```python
from build123d import *

# Parameters (mm, degrees)
BOSS_EXTRUDE1_OUTLINE_W = 13.462
BOSS_EXTRUDE1_OUTLINE_H = 19.685
BOSS_EXTRUDE1_OUTLINE_R = 2.159
BOSS_EXTRUDE1_DEPTH     = 2.54
SKETCH2_W               = 12.7
SKETCH2_H               = 19.685
SKETCH2_R               = 2.159
BOSS_EXTRUDE2_DEPTH     = 2.54
BOSS_EXTRUDE3_DEPTH     = 12.7
SKETCH4_R               = 1.9685
BOSS_EXTRUDE4_DEPTH     = 1.524


# Read off the part's stored shape, not the designer's step: Boss-Extrude1
with BuildPart() as part:
    # Boss-Extrude1 outline → Boss-Extrude1 (new body)
    with BuildSketch(Plane(origin=(0, 2.413, 0), x_dir=(1, 0, 0), z_dir=(0, 1, 0))):
        with Locations((-28.0035, 0)):
            Rectangle(BOSS_EXTRUDE1_OUTLINE_W, BOSS_EXTRUDE1_OUTLINE_H)
        with Locations((-24.511, -4.7625)):
            Circle(BOSS_EXTRUDE1_OUTLINE_R, mode=Mode.SUBTRACT)
        with Locations((-24.511, 4.7625)):
            Circle(BOSS_EXTRUDE1_OUTLINE_R, mode=Mode.SUBTRACT)
    extrude(amount=BOSS_EXTRUDE1_DEPTH)



with BuildPart() as body_2:
    # Sketch2 → Boss-Extrude2 (new body)
    with BuildSketch(Plane.XZ):
        with Locations((28.3845, 0)):
            Rectangle(SKETCH2_W, SKETCH2_H)
        with Locations(Location((24.511, 4.7625, 0), (0, 0, 270))):
            Circle(SKETCH2_R, mode=Mode.SUBTRACT)
        with Locations(Location((24.511, -4.7625, 0), (0, 0, 270))):
            Circle(SKETCH2_R, mode=Mode.SUBTRACT)
    extrude(amount=BOSS_EXTRUDE2_DEPTH)


with BuildPart() as part_1:
    add(part.part)

    add(body_2.part)  # Boss-Extrude3 merges body 2
    # Sketch3 → Boss-Extrude3 (add, symmetric)
    with BuildSketch(Plane.XY):
        Polygon((34.7345, -2.54), (34.7345, -30.988), (-34.7345, -30.988), (-34.7345, 2.413), (-32.1945, 2.413), (-32.1945, -28.448), (32.1945, -28.448), (32.1945, -2.54), align=None)
        Polygon((-32.1945, 4.953), (-32.1945, 26.884), (33.000418385, 26.884), (33.000418385, 29.424), (-34.7345, 29.424), (-34.7345, 4.953), align=None)
    extrude(amount=BOSS_EXTRUDE3_DEPTH, both=True)

    # Sketch4 → Boss-Extrude4 (add)
    with BuildSketch(Plane.XZ.offset(-26.884)):
        with Locations(Location((2.921, -8.382, 0), (0, 0, 90))):
            Circle(SKETCH4_R)
        with Locations(Location((19.685, -8.382, 0), (0, 0, 90))):
            Circle(SKETCH4_R)
        with Locations(Location((19.685, 8.382, 0), (0, 0, 90))):
            Circle(SKETCH4_R)
        with Locations(Location((2.921, 8.382, 0), (0, 0, 90))):
            Circle(SKETCH4_R)
    extrude(amount=BOSS_EXTRUDE4_DEPTH)


solid = part_1.part
```
The listing builds one solid part. Answer for the finished solid, in the listing's coordinates (mm). A direction names the side the tool comes from. Round coordinates to 2 decimals unless told otherwise and drop trailing zeros. Loops run counter-clockwise (first coordinate to the right, second up) from the corner with the lowest first, then second, coordinate; pieces in that order, holes last. Notation, with made-up numbers: (10, -26) - (66, -26) arc R14 cw to (66, -8) - close; hole circle Ø10 at (-25, -21.5). An arc over 180 degrees is marked (long way). Use one line per item in the form item = value. Start each with the question number.
1. Given pin 1 Ø1.5 at (y, z) = (16, -7.5) entering from +X; pin 2 Ø0.8 at (y, z) = (28.5, 3) entering from +X; pin 3 Ø12 at (x, y) = (17.5, 20.5) entering from -Z, each flat-ended and moving along its own axis, determine where each tip first touches the part or whether it passes through.
2. Consider line 1 (Y direction, x = 28, z = -8.5); line 2 (Y direction, x = -16.5, z = -7.5); line 3 (X direction, y = -4.5, z = -7). Determine where each line is inside the solid, lowest interval first. Write a range as [from, to].
3. The part is cut by section C-C on x = 28. Determine the outline of the cut face in (y, z), then the cut area to 3 significant figures.
4. The part is cut by section B-B on x = -12. Determine the outline of the cut face in (y, z).
5. The part is cut by section A-A on y = -14.5. Determine the outline of the cut face in (x, z), then the cut area to 3 significant figures.
6. For a pull along X with two mould halves and no side action, classify faces 4 (the face through (22.403, -1.252, 5.231)), 5 (the face through (-26.102, 3.665, -6.222)), 6 (the face through (3, 25.36, 8)), 7 (the face through (-34.734, 0, 0)) as pulls with the +X half, pulls with the -X half, needs draft (parallel to the pull), parting line crosses it, or undercut.
7. The part is cut by section D-D on y = -1. Determine the outline of the cut face in (x, z).
8. A tool of negligible diameter and unlimited length cuts with its end or side. For faces 1 (the face through (-21.272, 4, 0)), 2 (the face through (-28, 4, -9.842)), 3 (the face through (2.33, 26.13, 10.26)), from which of +Z, -Z, +X, -X, +Y, -Y can it reach the whole face along a straight path? Write none if from no direction.
Geometry check:
q1.pin_1 = -32.19
q1.pin_2 = 33
q1.pin_3 = -10.35
q2.line_1 = [-30.99, -28.45], [-2.54, 0], [26.88, 29.42]
q2.line_2 = [-30.99, -28.45], [26.88, 29.42]
q2.line_3 = [-34.73, -32.19], [32.19, 34.73]
q3.outline = (-30.99, -12.7) - (-28.45, -12.7) - (-28.45, 12.7) - (-30.99, 12.7) - close; (-2.54, -9.84) - (0, -9.84) - (0, 9.84) - (-2.54, 9.84) - close; (26.88, -12.7) - (29.42, -12.7) - (29.42, 12.7) - (26.88, 12.7) - close
q3.area = 179 mm^2
q4.outline = (-30.99, -12.7) - (-28.45, -12.7) - (-28.45, 12.7) - (-30.99, 12.7) - close; (26.88, -12.7) - (29.42, -12.7) - (29.42, 12.7) - (26.88, 12.7) - close
q5.outline = (-34.73, -12.7) - (-32.19, -12.7) - (-32.19, 12.7) - (-34.73, 12.7) - close; (32.19, -12.7) - (34.73, -12.7) - (34.73, 12.7) - (32.19, 12.7) - close
q5.area = 129 mm^2
q6.face_4 = undercut
q6.face_5 = undercut
q6.face_6 = needs draft
q6.face_7 = pulls with the -X half
q7.outline = (-34.73, -12.7) - (-32.19, -12.7) - (-32.19, 12.7) - (-34.73, 12.7) - close; (22.03, -9.84) - (34.73, -9.84) - (34.73, 9.84) - (22.03, 9.84) - close; hole circle Ø4.32 at (24.51, -4.76); hole circle Ø4.32 at (24.51, 4.76)
q8.face_1 = +Z, -Z, +X
q8.face_2 = -Z, +X, -X
q8.face_3 = none
